from build123d import *

# Parameters (mm, degrees)
SKETCH_1_R      = 6.5
EXTRUDE_1_DEPTH = 0.5
SKETCH_2_R      = 7.75
EXTRUDE_2_DEPTH = 2.5
SKETCH_3_R      = 9
EXTRUDE_3_DEPTH = 2
SKETCH_4_R      = 14.25
EXTRUDE_4_DEPTH = 1
SKETCH_5_R      = 14.25
SKETCH_5_R_2    = 13.5
EXTRUDE_5_DEPTH = 3


with BuildPart() as part:
    # Эскиз1 → Бобышка-Вытянуть1 (new body)
    with BuildSketch(Plane.XY):
        Circle(SKETCH_1_R)
    extrude(amount=EXTRUDE_1_DEPTH)

    # Эскиз2 → Бобышка-Вытянуть2 (add)
    with BuildSketch(Plane.XY.offset(0.5)):
        Circle(SKETCH_2_R)
    extrude(amount=EXTRUDE_2_DEPTH)

    # Эскиз3 → Бобышка-Вытянуть3 (add)
    with BuildSketch(Plane.XY.offset(3)):
        Circle(SKETCH_3_R)
    extrude(amount=EXTRUDE_3_DEPTH)

    # Эскиз4 → Бобышка-Вытянуть4 (add)
    with BuildSketch(Plane.XY.offset(5)):
        Circle(SKETCH_4_R)
    extrude(amount=EXTRUDE_4_DEPTH)

    # Эскиз5 → Бобышка-Вытянуть5 (add)
    with BuildSketch(Plane.XY.offset(6)):
        Circle(SKETCH_5_R)
        Circle(SKETCH_5_R_2, mode=Mode.SUBTRACT)
    extrude(amount=EXTRUDE_5_DEPTH)


solid = part.part
The model under review builds one solid part; all positions refer to its coordinate system, in mm. A direction names the side the tool comes from. Round coordinates to 2 decimals unless told otherwise and drop trailing zeros. Order: outer loops, then holes, each group sorted by start corner. A loop starts at its lowest first (then second) coordinate and runs counter-clockwise, first axis right, second up. Notation, with made-up numbers: (66, 43.25) -> (75, 43.25) arc R17 ccw to (75, 62.25) -> close; hole circle Ø3 at (33, 40.5). An arc over 180 degrees is marked (long way). Return JSON: item names as keys, results as strings.
1. For faces 4 (the face through (13, -5, 9)), 5 (the face through (-5.158, -3.955, 0.246)), 6 (the face through (-2.93, -13.18, 7.48)), list the 3-axis set-ups (+Z, -Z, +X, -X, +Y, -Y) from which the entire face can be reached by the end or side of a thin tool; tool diameter is ignored.
Answer block:
{"face 4": "+Z, +X, -X, +Y, -Y", "face 5": "-Z", "face 6": "+Z"}
2. Take a section at D-D (z = 4). Write out the cut boundary in (x, y).
Answer block:
{"outline": "circle Ø18 at (0, 0)"}
3. Insertion check: P1, Ø8, axis at x = -4.5, y = -1, coming from the +Z side; P2, Ø1, axis at y = -3.5, z = 3, coming from the -X side; P3, Ø5, axis at y = 3, z = 4, coming from the -X side; P4, Ø1, axis at y = -9.5, z = 1.5, coming from the -X side. Each pin has a flat end and moves straight along its axis. Give the tip position at first contact, or say it passes through.
Answer block:
{"P1": "stops at z = 6", "P2": "stops at x = -8.49", "P3": "stops at x = -14.23", "P4": "passes through"}
4. For L1, parallel to Y at x = 0, z = 7.25; L2, parallel to Z at x = 5, y = 12.25; L3, parallel to Z at x = -5, y = 5.25, list the stretches that pass through material, from the lowest coordinate up. Write a range as [from, to].
Answer block:
{"L1": "y = [-14.25, -13.5], [13.5, 14.25]", "L2": "z = [5, 6]", "L3": "z = [0.5, 6]"}
5. Take a section at B-B (z = 7). Write out the cut boundary in (x, y), then the cut area to 3 significant figures.
Answer block:
{"outline": "circle Ø28.5 at (0, 0); hole circle Ø27 at (0, 0)", "area": "65.4 mm²"}
6. The part is to be moulded in two halves that separate along Y. For faces 1 (the face through (13.163, -5.458, 6.972)), 2 (the face through (0, 0, 6)), 3 (the face through (0, 0, 0)), say which applies: +Y half, -Y half, draft (parallel to the pull), parting line (faces both ways), or undercut.
Answer block:
{"face 1": "parting line", "face 2": "undercut", "face 3": "draft"}
7. Take a section at A-A (y = 0). Write out the cut boundary in (x, z), then the cut area to 3 significant figures.
Answer block:
{"outline": "(-14.25, 5) -> (-9, 5) -> (-9, 3) -> (-7.75, 3) -> (-7.75, 0.5) -> (-6.5, 0.5) -> (-6.5, 0) -> (6.5, 0) -> (6.5, 0.5) -> (7.75, 0.5) -> (7.75, 3) -> (9, 3) -> (9, 5) -> (14.25, 5) -> (14.25, 9) -> (13.5, 9) -> (13.5, 6) -> (-13.5, 6) -> (-13.5, 9) -> (-14.25, 9) -> close", "area": "114 mm²"}
